Input: part model. Units: mm. Frame: model coordinates. A direction names the side the tool comes from. Coordinates: 2 decimals unless noted, no trailing zeros. Order: outer loops, then holes, each group sorted by start corner. A loop starts at its lowest first (then second) coordinate and runs counter-clockwise, first axis right, second up. Notation, with made-up numbers: M -35,16 L -20,16 A25 ccw -20,34 Z; hole C 40,61.5 d8. An arc over 180 degrees is marked long. Answer in a Markdown table with one row per item.
from build123d import *

# Parameters (mm, degrees)
SKETCH1_R           = 40
BOSS_EXTRUDE1_DEPTH = 3
SKETCH3_R           = 32.5
BOSS_EXTRUDE2_DEPTH = 15
SKETCH4_R           = 2.82527212
CUT_EXTRUDE1_DEPTH  = 60.363288319
SKETCH5_R           = 11.6
CUT_EXTRUDE2_DEPTH  = 60.363288319


with BuildPart() as part:
    # Sketch1 → Boss-Extrude1 (new body)
    with BuildSketch(Plane(origin=(0, 0, 0), x_dir=(1, 0, 0), z_dir=(0, 1, 0))):
        with Locations(Location((0, 0, 0), (0, 0, 270))):
            Circle(SKETCH1_R)
    extrude(amount=BOSS_EXTRUDE1_DEPTH)

    # Sketch3 → Boss-Extrude2 (add)
    with BuildSketch(Plane(origin=(0, 3, 0), x_dir=(1, 0, 0), z_dir=(0, 1, 0))):
        with Locations(Location((0, 0, 0), (0, 0, 270))):
            Circle(SKETCH3_R)
    extrude(amount=BOSS_EXTRUDE2_DEPTH)

    # Sketch4 → Cut-Extrude1 (cut, through all)
    with BuildSketch(Plane(origin=(0, 18, 0), x_dir=(1, 0, 0), z_dir=(0, 1, 0))):
        with Locations(Location((0, 22.5, 0), (0, 0, 270))):
            Circle(SKETCH4_R)
        with Locations(Location((15.909902577, 15.909902577, 0), (0, 0, 270))):
            Circle(SKETCH4_R)
        with Locations(Location((22.5, 0, 0), (0, 0, 270))):
            Circle(SKETCH4_R)
        with Locations(Location((15.909902577, -15.909902577, 0), (0, 0, 270))):
            Circle(SKETCH4_R)
        with Locations(Location((0, -22.5, 0), (0, 0, 270))):
            Circle(SKETCH4_R)
        with Locations(Location((-15.909902577, -15.909902577, 0), (0, 0, 270))):
            Circle(SKETCH4_R)
        with Locations(Location((-22.5, 0, 0), (0, 0, 270))):
            Circle(SKETCH4_R)
        with Locations(Location((-15.909902577, 15.909902577, 0), (0, 0, 270))):
            Circle(SKETCH4_R)
    extrude(amount=-CUT_EXTRUDE1_DEPTH, mode=Mode.SUBTRACT)

    # Sketch5 → Cut-Extrude2 (cut, through all)
    with BuildSketch(Plane.XZ):
        with Locations(Location((0, 0, 0), (0, 0, 270))):
            Circle(SKETCH5_R)
    extrude(amount=-CUT_EXTRUDE2_DEPTH, mode=Mode.SUBTRACT)


solid = part.part
1) Contact query for flat-ended pins moving along their axis: pin 1 (4 mm diameter, centred on x = -32, z = 15.5, fed in from +Y); pin 2 (2 mm diameter, centred on x = 5.5, y = 11, fed in from -Z); pin 3 (8 mm diameter, centred on x = 8, y = 14, fed in from +Z). Output: stop coordinate, or through.
Resolved:
| item | result |
|---|---|
| pin 1 | stops at y = 3 |
| pin 2 | stops at z = -32.19 |
| pin 3 | stops at z = 32.25 |
2) Cut plane A-A, the plane z = 0. Output: boundary loops of the cut face in (x, y).
Resolved:
| item | result |
|---|---|
| outline | M -40,0 L -25.33,0 L -25.33,18 L -32.5,18 L -32.5,3 L -40,3 Z; M -19.67,0 L -11.6,0 L -11.6,18 L -19.67,18 Z; M 11.6,0 L 19.67,0 L 19.67,18 L 11.6,18 Z; M 25.33,0 L 40,0 L 40,3 L 32.5,3 L 32.5,18 L 25.33,18 Z |
3) Material intervals for probe 1 along X at (y, z) = (13.25, 0); probe 2 along Z at (x, y) = (15.5, 8); probe 3 along Y at (x, z) = (-30.5, -22.5), sorted ascending.
Resolved:
| item | result |
|---|---|
| probe 1 | x = -32.5 to -25.33, -19.67 to -11.6, 11.6 to 19.67, 25.33 to 32.5 |
| probe 2 | z = -28.57 to -18.71, -13.11 to 13.11, 18.71 to 28.57 |
| probe 3 | y = 0 to 3 |
4) Cut plane B-B, the plane x = -1. Output: boundary loops of the cut face in (y, z).
Resolved:
| item | result |
|---|---|
| outline | M 0,-39.99 L 3,-39.99 L 3,-32.48 L 18,-32.48 L 18,-25.14 L 0,-25.14 Z; M 0,-19.86 L 18,-19.86 L 18,-11.56 L 0,-11.56 Z; M 0,11.56 L 18,11.56 L 18,19.86 L 0,19.86 Z; M 0,25.14 L 18,25.14 L 18,32.48 L 3,32.48 L 3,39.99 L 0,39.99 Z |
5) Mould query, pull axis X, two halves, no side actions, for faces 1 (the face through (0, 18, 14)), 2 (the face through (0.124, 9.126, -25.323)), 3 (the face through (9.76, 10.4, 31)). Classes: +X half, -X half, draft (parallel to the pull), parting line (faces both ways), or undercut.
Resolved:
| item | result |
|---|---|
| face 1 | draft |
| face 2 | undercut |
| face 3 | parting line |
6) Reachability of faces 4 (the face through (-13.11, 9.13, 15.54)), 5 (the face through (33, 3, 0)) from +Z, -Z, +X, -X, +Y, -Y: full face, straight path, thin tool, end or side. Return the list, or none.
Resolved:
| item | result |
|---|---|
| face 4 | +Y, -Y |
| face 5 | +Y |
7) Cut plane D-D, the plane x = -14.5. Output: boundary loops of the cut face in (y, z), and give its area (3 significant figures).
Resolved:
| item | result |
|---|---|
| outline | M 0,-37.28 L 3,-37.28 L 3,-29.09 L 18,-29.09 L 18,-18.36 L 0,-18.36 Z; M 0,-13.46 L 18,-13.46 L 18,13.46 L 0,13.46 Z; M 0,18.36 L 18,18.36 L 18,29.09 L 3,29.09 L 3,37.28 L 0,37.28 Z |
| area | 920 mm2 |
8) Cut plane C-C, the plane y = 5.5. State how many separate pieces and enclosed holes the cut face has, and give its area (3 significant figures).
Resolved:
| item | result |
|---|---|
| separate pieces | 1 |
| enclosed holes | 9 |
| area | 2,690 mm2 |
